```python
from build123d import *

# Parameters (mm, degrees)
F4_DEPTH = 12.7
F5_R     = 6.1731972722
F6_DEPTH = 12.7
F7_DEPTH = 12.7


# Not quite as in the source:
# - a feature of the source that left no trace in its solid (it failed there, or was rolled back) is left out


with BuildPart() as f4:
    # F3 (on Top) → F4 (new body)
    with BuildSketch(Plane.XY):
        with BuildLine():
            Line((-247.0177412033, 0), (-247.0177412033, 27.8642479823))
            ThreePointArc((-247.0177412033, 27.8642479823), (-274.8819891856, 0), (-247.0177412033, -27.8642479823))
            Line((-247.0177412033, -27.8642479823), (-247.0177412033, 0))
        make_face()
    extrude(amount=F4_DEPTH)

    # F5 (on face) → F6 (join)
    with BuildSketch(Plane.XY.offset(12.7)):
        with Locations((-258.7949037552, 0)):
            Circle(F5_R)
    extrude(amount=-F6_DEPTH)

    # F5 (on face) → F7 (join)
    with BuildSketch(Plane.XY.offset(12.7)):
        with Locations((-258.7949037552, 0)):
            Circle(F5_R)
    extrude(amount=-F7_DEPTH)


solid = f4.part
```
Could you check a few things on this model? Use its own coordinates, in mm. Round coordinates to 2 decimals unless told otherwise and drop trailing zeros. Write each loop counter-clockwise with the first axis right and the second up, starting at its lowest first coordinate (ties: lowest second). Pieces come first, ordered by that corner, then holes. Notation, with made-up numbers: M 64.5,21 L 79.5,21 A14 ccw 79.5,35 Z; hole C 39,11 d6. An arc over 180 degrees is marked long. Answer in a Markdown table with one row per item. Add a question column.
Q1. Imagine slicing it at C-C (x = -265.5). Please give me the cut outline in (y, z).
Q2. Imagine slicing it at B-B (y = 11.5). Please give me the cut outline in (x, z), then the cut area to 3 significant figures.
Q3. Will these pins go through, and if not, where does the flat tip stop? pin 1 Ø6 at (y, z) = (-18, 5.5) entering from -X; pin 2 Ø2 at (y, z) = (10.5, 9.5) entering from -X; pin 3 Ø4 at (x, z) = (-250.5, 8.5) entering from +Y.
Q4. If I drill on line 1 (X direction, y = 0, z = 1); line 2 (Y direction, x = -268, z = 0.75); line 3 (X direction, y = -2, z = 9), over which ranges is the centre line in solid material (lowest first)? Write a range as from..to.
Q5. Imagine slicing it at A-A (z = 9.5). Please give me the cut outline in (x, y).
Values:
| question | item | result |
|---|---|---|
| 1 | outline | M -20.85,0 L 20.85,0 L 20.85,12.7 L -20.85,12.7 Z |
| 2 | outline | M -272.4,0 L -247.02,0 L -247.02,12.7 L -272.4,12.7 Z |
| 2 | area | 322 mm^2 |
| 3 | pin 1 | x = -270.5 |
| 3 | pin 2 | x = -273.21 |
| 3 | pin 3 | y = 27.82 |
| 4 | line 1 | -274.88..-247.02 |
| 4 | line 2 | -18.33..18.33 |
| 4 | line 3 | -274.81..-247.02 |
| 5 | outline | M -247.02,-27.86 L -247.02,27.86 A27.86 ccw Z |
